from build123d import *

# Parameters (mm, degrees)
BOSS_EXTRUDE4_DEPTH = 8
SKETCH2_R           = 2.5
CUT_EXTRUDE1_DEPTH  = 5.15


with BuildPart() as part:
    # Sketch1 → Boss-Extrude4 (new body)
    with BuildSketch(Plane(origin=(0, 0, 0), x_dir=(1, 0, 0), z_dir=(0, 1, 0))):
        with BuildLine():
            Line((-4.119957175, -14.5), (4.119957175, -14.5))
            ThreePointArc((4.119957175, -14.5), (4.42252042, -14.398064672), (4.60171613, -14.133821932))
            Line((4.60171613, -14.133821932), (6.638196956, -6.80249096))
            ThreePointArc((6.638196956, -6.80249096), (6.871082847, -5.489641243), (6.850811782, -4.156449845))
            Line((6.850811782, -4.156449845), (4.720984417, 15.024219546))
            ThreePointArc((4.720984417, 15.024219546), (0, 19.25), (-4.720984417, 15.024219546))
            Line((-4.720984417, 15.024219546), (-6.850811782, -4.156449845))
            ThreePointArc((-6.850811782, -4.156449845), (-6.871082847, -5.489641243), (-6.638196956, -6.80249096))
            Line((-6.638196956, -6.80249096), (-4.60171613, -14.133821932))
            ThreePointArc((-4.60171613, -14.133821932), (-4.42252042, -14.398064672), (-4.119957175, -14.5))
        make_face()
    extrude(amount=BOSS_EXTRUDE4_DEPTH)

    # Sketch2 → Cut-Extrude1 (cut)
    with BuildSketch(Plane(origin=(0, 8, 0), x_dir=(1, 0, 0), z_dir=(0, 1, 0))):
        with Locations(Location((-0.106428412, -4.928983913, 0), (0, 0, 270))):
            Circle(SKETCH2_R)
    extrude(amount=-CUT_EXTRUDE1_DEPTH, mode=Mode.SUBTRACT)


solid = part.part
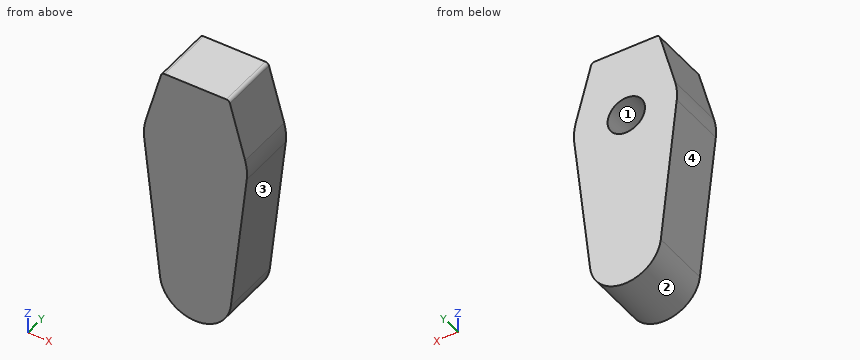
Check sheet for the modelled part. Datum: model origin and axes. Units: mm. Face numbers are marked on the shaded views. Give positions to 0.01 mm unless a question says otherwise; leave off trailing zeros. Write each loop counter-clockwise with the first axis right and the second up, starting at its lowest first coordinate (ties: lowest second). Pieces come first, ordered by that corner, then holes. Notation, with made-up numbers: (41, 0) -> (92, 0) arc R24 ccw to (92, 21) -> close; hole circle Ø6 at (35, 21.5). An arc over 180 degrees is marked (long way). One line per item, written item: value. Start each with the question number.
Item 1: Section check D-D on x = 3.75. Record the cut outline in (y, z).
Item 2: Section check B-B on x = 0.5. Record the cut outline in (y, z).
Item 3: Gauge pin test, flat ends, axial feed: pin 1 (4 mm diameter, centred on x = 3.5, y = 2.5, fed in from -Z); pin 2 (1.5 mm diameter, centred on x = -0.5, z = 4.5, fed in from +Y); pin 3 (3 mm diameter, centred on y = 6, z = 11, fed in from -X). Record the tip position at first contact, or that the pin passes through.
Item 4: Draft check along X on the marked faces 1, 2, 3 and 4. Enter one of: +X half, -X half, draft (parallel to the pull), parting line (faces both ways), or undercut.
Item 5: Section check A-A on y = 2.25. Record the cut outline in (x, z), then the cut area to 3 significant figures.
Item 6: Material ranges on probe 1 along X at (y, z) = (3.75, 7); probe 2 along Z at (x, y) = (-1.25, 6.25); probe 3 along X at (y, z) = (6, 4.5), recorded low to high. Write a range as from..to.
Item 7: Section check C-C on z = -9.5. Record the cut outline in (x, y).
Results list:
1. outline: (0, -17.42) -> (8, -17.42) -> (8, 14.5) -> (0, 14.5) -> close
2. outline: (0, -19.22) -> (8, -19.22) -> (8, 2.5) -> (2.85, 2.5) -> (2.85, 7.35) -> (8, 7.35) -> (8, 14.5) -> (0, 14.5) -> close
3. pin 1: z = -19.01
3. pin 2: y = 2.85
3. pin 3: x = -5.89
4. face 1: undercut
4. face 2: parting line
4. face 3: +X half
4. face 4: -X half
5. outline: (-6.85, 4.16) -> (-4.72, -15.02) arc R4.75 ccw to (4.72, -15.02) -> (6.85, 4.16) arc R7 ccw to (6.64, 6.8) -> (4.6, 14.13) arc R0.5 ccw to (4.12, 14.5) -> (-4.12, 14.5) arc R0.5 ccw to (-4.6, 14.13) -> (-6.64, 6.8) arc R7 ccw to start
5. area: 374 mm²
6. probe 1: -6.58..-1.51, 1.29..6.58
6. probe 2: -19.08..2.71, 7.15..14.5
6. probe 3: -6.88..-2.57, 2.36..6.88
7. outline: (-5.33, 0) -> (5.33, 0) -> (5.33, 8) -> (-5.33, 8) -> close
